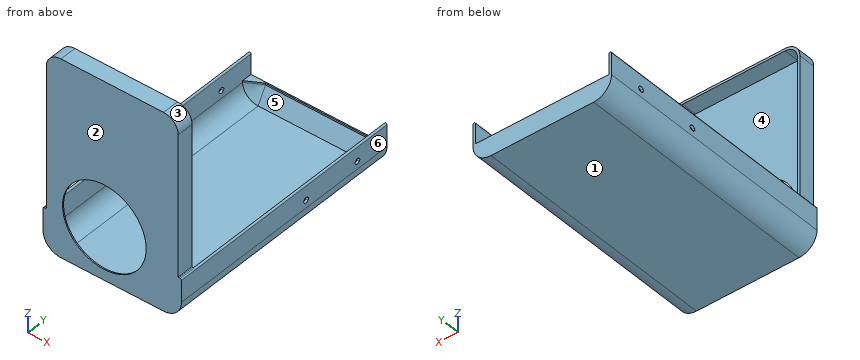
```python
from build123d import *
from OCP.BRepFilletAPI import BRepFilletAPI_MakeChamfer

# Parameters (mm, degrees)
BOSS_EXTRUDE1_DEPTH = 160
BOSS_EXTRUDE2_START = -0.8
BOSS_EXTRUDE2_DEPTH = 0.8
CUT_EXTRUDE1_DEPTH  = 185.952426316
SKETCH4_R           = 27
BOSS_EXTRUDE3_DEPTH = 0.8
FILLET1_R           = 0.4
BOSS_EXTRUDE4_DEPTH = 10
FILLET2_R           = 2
CHAMFER1_SIZE       = 5.7
CHAMFER1_SIZE2      = 9.872689603


with BuildPart() as part:
    # Sketch1 → Boss-Extrude1 (new body)
    with BuildSketch(Plane(origin=(0, 0, 0), x_dir=(1, 0, 0), z_dir=(0, 1, 0))):
        with BuildLine():
            Line((-33.1, 0), (33.1, 0))
            ThreePointArc((33.1, 0), (40.171067812, -2.928932188), (43.1, -10))
            Line((43.1, -10), (43.1, -24))
            ThreePointArc((43.1, -24), (43.9, -24.8), (44.7, -24))
            Line((44.7, -24), (44.7, -10))
            ThreePointArc((44.7, -10), (41.302438662, -1.797561338), (33.1, 1.6))
            Line((33.1, 1.6), (-33.1, 1.6))
            ThreePointArc((-33.1, 1.6), (-41.302438662, -1.797561338), (-44.7, -10))
            Line((-44.7, -10), (-44.7, -24))
            ThreePointArc((-44.7, -24), (-43.9, -24.8), (-43.1, -24))
            Line((-43.1, -24), (-43.1, -10))
            ThreePointArc((-43.1, -10), (-40.171067812, -2.928932188), (-33.1, 0))
        make_face()
    extrude(amount=BOSS_EXTRUDE1_DEPTH)

    # Sketch2 → Boss-Extrude2 (add)
    with BuildSketch(Plane(origin=(0, 160, 0), x_dir=(1, 0, 0), z_dir=(0, 1, 0)).offset(BOSS_EXTRUDE2_START)):
        with BuildLine():
            Line((44.7, -10), (44.7, -11))
            Line((44.7, -11), (-44.7, -11))
            Line((-44.7, -11), (-44.7, -10))
            ThreePointArc((-44.7, -10), (-41.302438662, -1.797561338), (-33.1, 1.6))
            Line((-33.1, 1.6), (33.1, 1.6))
            ThreePointArc((33.1, 1.6), (41.302438662, -1.797561338), (44.7, -10))
        make_face()
    extrude(amount=BOSS_EXTRUDE2_DEPTH)

    # Sketch3 → Cut-Extrude1 (cut, through all)
    with BuildSketch(Plane(origin=(44.7, 0, 0), x_dir=(0, 0, -1), z_dir=(1, 0, 0))):
        with BuildLine():
            Line((-15.875, 138.515544457), (-15, 139.020725942))
            Line((-15, 139.020725942), (-14.125, 138.515544457))
            ThreePointArc((-14.125, 138.515544457), (-13.25, 137), (-14.125, 135.484455543))
            Line((-14.125, 135.484455543), (-15, 134.979274058))
            Line((-15, 134.979274058), (-15.875, 135.484455543))
            ThreePointArc((-15.875, 135.484455543), (-16.75, 137), (-15.875, 138.515544457))
        make_face()
        with BuildLine():
            Line((-15.875, 98.515544457), (-15, 99.020725942))
            Line((-15, 99.020725942), (-14.125, 98.515544457))
            ThreePointArc((-14.125, 98.515544457), (-13.25, 97), (-14.125, 95.484455543))
            Line((-14.125, 95.484455543), (-15, 94.979274058))
            Line((-15, 94.979274058), (-15.875, 95.484455543))
            ThreePointArc((-15.875, 95.484455543), (-16.75, 97), (-15.875, 98.515544457))
        make_face()
    extrude(amount=-CUT_EXTRUDE1_DEPTH, mode=Mode.SUBTRACT)

    # Sketch4 → Boss-Extrude3 (add)
    with BuildSketch(Plane.XZ):
        with BuildLine():
            Line((-43.9, 24.8), (-42.6, 24.8))
            Line((-42.6, 24.8), (-42.6, 115.8))
            ThreePointArc((-42.6, 115.8), (-39.817514421, 122.517514421), (-33.1, 125.3))
            Line((-33.1, 125.3), (33.1, 125.3))
            ThreePointArc((33.1, 125.3), (39.817514421, 122.517514421), (42.6, 115.8))
            Line((42.6, 115.8), (42.6, 24.8))
            Line((42.6, 24.8), (43.9, 24.8))
            ThreePointArc((43.9, 24.8), (43.334314575, 24.565685425), (43.1, 24))
            Line((43.1, 24), (43.1, 10))
            ThreePointArc((43.1, 10), (40.171067812, 2.928932188), (33.1, 0))
            Line((33.1, 0), (-33.1, 0))
            ThreePointArc((-33.1, 0), (-40.171067812, 2.928932188), (-43.1, 10))
            Line((-43.1, 10), (-43.1, 24))
            ThreePointArc((-43.1, 24), (-43.334314575, 24.565685425), (-43.9, 24.8))
        make_face()
        with Locations(Location((-5.1, 32.3, 0), (0, 0, 270))):
            Circle(SKETCH4_R, mode=Mode.SUBTRACT)
    extrude(amount=-BOSS_EXTRUDE3_DEPTH)

    # Fillet1
    fillet1_edges = [part.edges().sort_by_distance(p)[0] for p in [
        (-42.6, 0.4, 24.8),
        (42.6, 0.4, 24.8),
    ]]
    fillet(fillet1_edges, radius=FILLET1_R)

    # Sketch6 → Boss-Extrude4 (add)
    with BuildSketch(Plane(origin=(0, 0.8, 0), x_dir=(1, 0, 0), z_dir=(0, 1, 0))):
        with BuildLine():
            Line((-43.1, -23.2), (-43, -23.2))
            ThreePointArc((-43, -23.2), (-41.585786438, -23.785786438), (-41, -25.2))
            Line((-41, -25.2), (-41, -115.8))
            ThreePointArc((-41, -115.8), (-38.686143571, -121.386143571), (-33.1, -123.7))
            Line((-33.1, -123.7), (33.1, -123.7))
            ThreePointArc((33.1, -123.7), (38.686143571, -121.386143571), (41, -115.8))
            Line((41, -115.8), (41, -25.2))
            ThreePointArc((41, -25.2), (41.585786438, -23.785786438), (43, -23.2))
            Line((43, -23.2), (43.1, -23.2))
            Line((43.1, -23.2), (43.1, -24))
            ThreePointArc((43.1, -24), (43.334314575, -24.565685425), (43.9, -24.8))
            Line((43.9, -24.8), (43, -24.8))
            ThreePointArc((43, -24.8), (42.717157288, -24.917157288), (42.6, -25.2))
            Line((42.6, -25.2), (42.6, -115.8))
            ThreePointArc((42.6, -115.8), (39.817514421, -122.517514421), (33.1, -125.3))
            Line((33.1, -125.3), (-33.1, -125.3))
            ThreePointArc((-33.1, -125.3), (-39.817514421, -122.517514421), (-42.6, -115.8))
            Line((-42.6, -115.8), (-42.6, -25.2))
            ThreePointArc((-42.6, -25.2), (-42.717157288, -24.917157288), (-43, -24.8))
            Line((-43, -24.8), (-43.9, -24.8))
            ThreePointArc((-43.9, -24.8), (-43.334314575, -24.565685425), (-43.1, -24))
            Line((-43.1, -24), (-43.1, -23.2))
        make_face()
    extrude(amount=BOSS_EXTRUDE4_DEPTH)

    # Fillet2
    # the kernel refuses this fillet: 2 mm, written as the material it adds along each edge
    with BuildSketch(Plane(origin=(43.1, 0.8, 23.2), x_dir=(-0.9748527767632401, 0, 0.22284986793130537), z_dir=(0, 1, 0))) as fillet2_piece_1:
        with BuildLine():
            CenterArc((1.610986416, -1.927420567), FILLET2_R, 105.482875224, 61.640649972)
            Line((-0.338719137, -1.481720831), (-0.533689693, -1.437150857))
            Line((-0.533689693, -1.437150857), (-0.194970555, 0.044569974))
            Line((-0.194970555, 0.044569974), (0.044569974, 0.194970555))
            ThreePointArc((0.044569974, 0.194970555), (0.142055251, 0.172685569), (1.023695645, 0.192742057))
            Line((1.023695645, 0.192742057), (1.077085715, 0))
        make_face()
    extrude(amount=10)
    with BuildSketch(Plane(origin=(-43.1, 0.8, 23.2), x_dir=(0.9748527767632457, 0, 0.2228498679312814), z_dir=(0, 1, 0))) as fillet2_piece_2:
        with BuildLine():
            CenterArc((1.610986416, 1.927420567), FILLET2_R, 192.876474804, 61.640649972)
            Line((-0.338719137, 1.481720831), (-0.533689693, 1.437150857))
            Line((-0.533689693, 1.437150857), (-0.194970555, -0.044569974))
            Line((-0.194970555, -0.044569974), (0.044569974, -0.194970555))
            ThreePointArc((0.044569974, -0.194970555), (0.142055251, -0.172685569), (1.023695645, -0.192742057))
            Line((1.023695645, -0.192742057), (1.077085715, 0))
        make_face()
    extrude(amount=10)

    # Chamfer1: one chamfer whose edges measure the first distance from different faces: ONE call of the kernel's chamfer builder (chamfer() names one face for all edges)
    chamfer1_edges_1 = [part.edges().sort_by_distance(p)[0] for p in [
        (0, 159.2, 0),
    ]]
    chamfer1_side_1 = [part.faces().sort_by_distance(p)[0] for p in [
        (0, 80, 0),
    ]]
    chamfer1_edges_2 = [part.edges().sort_by_distance(p)[0] for p in [
        (40.171067812, 159.2, 2.928932188),
    ]]
    chamfer1_side_2 = [part.faces().sort_by_distance(p)[0] for p in [
        (40.171067812, 80, 2.928932188),
    ]]
    chamfer1_edges_3 = [part.edges().sort_by_distance(p)[0] for p in [
        (43.1, 159.2, 10.5),
    ]]
    chamfer1_side_3 = [part.faces().sort_by_distance(p)[0] for p in [
        (43.1, 80.829745828, 16.958586697),
    ]]
    chamfer1_edges_4 = [part.edges().sort_by_distance(p)[0] for p in [
        (-43.1, 159.2, 10.5),
    ]]
    chamfer1_side_4 = [part.faces().sort_by_distance(p)[0] for p in [
        (-43.1, 80.829745828, 16.958586697),
    ]]
    chamfer1_edges_5 = [part.edges().sort_by_distance(p)[0] for p in [
        (-40.171067812, 159.2, 2.928932188),
    ]]
    chamfer1_side_5 = [part.faces().sort_by_distance(p)[0] for p in [
        (-40.171067812, 80, 2.928932188),
    ]]
    chamfer1 = BRepFilletAPI_MakeChamfer(part.part.solid().wrapped)
    for e in chamfer1_edges_1:
        chamfer1.Add(CHAMFER1_SIZE, CHAMFER1_SIZE2, e.wrapped, chamfer1_side_1[0].wrapped)  # the first distance lies on this face
    for e in chamfer1_edges_2:
        chamfer1.Add(CHAMFER1_SIZE, CHAMFER1_SIZE2, e.wrapped, chamfer1_side_2[0].wrapped)  # the first distance lies on this face
    for e in chamfer1_edges_3:
        chamfer1.Add(CHAMFER1_SIZE, CHAMFER1_SIZE2, e.wrapped, chamfer1_side_3[0].wrapped)  # the first distance lies on this face
    for e in chamfer1_edges_4:
        chamfer1.Add(CHAMFER1_SIZE, CHAMFER1_SIZE2, e.wrapped, chamfer1_side_4[0].wrapped)  # the first distance lies on this face
    for e in chamfer1_edges_5:
        chamfer1.Add(CHAMFER1_SIZE, CHAMFER1_SIZE2, e.wrapped, chamfer1_side_5[0].wrapped)  # the first distance lies on this face
    add(Compound.cast(chamfer1.Shape()), mode=Mode.REPLACE)


solid = part.part
```
CAD build for the part. Positions are in the model's coordinates, mm. Face numbers are marked on the shaded views. A direction names the side the tool comes from. Give positions to 0.01 mm unless a question says otherwise; leave off trailing zeros. Order: outer loops, then holes, each group sorted by start corner. A loop starts at its lowest first (then second) coordinate and runs counter-clockwise, first axis right, second up.
(1) Tool access for the marked faces 5 and 6: list every direction of +Z, -Z, +X, -X, +Y, -Y with a clear straight run to the whole face (end or side of a thin tool).
(2) Saw through at C-C, the plane z = 77. Give the cut face in (x, y), then the cut area to 3 significant figures.
(3) Saw through at B-B, the plane x = -5.1. Give the cut face in (y, z).
(4) Flat gauge pins, fed straight in: pin 1 (1.5 mm diameter, centred on x = 0, y = 45, fed in from +Z); pin 2 (5.5 mm diameter, centred on y = 6.5, z = 85, fed in from +X); pin 3 (5 mm diameter, centred on y = 4, z = 82, fed in from -X). Where does each tip first touch, or does it go through?
(5) Drill centre lines: L1, parallel to Z at x = 23.5, y = 9.5; L2, parallel to X at y = 0.65, z = 32.3; L3, parallel to X at y = 94, z = 18. Where is each one in solid material? Low to high.
(6) Mould opens along Z. For the marked faces 1, 2, 3 and 4 say: released by +Z, released by -Z, zero draft, split by the parting line, or undercut.
(7) Saw through at A-A, the plane z = 32.3. Give the cut face in (x, y), then the cut area to 3 significant figures.
(8) Saw through at D-D, the plane y = 47. Give the cut face in (x, z), then the cut area to 3 significant figures.
Results found:
1. face 5: +Z
1. face 6: +Z, -Z, +X, +Y, -Y
2. outline: (-42.6, 0) - (42.6, 0) - (42.6, 10.8) - (41, 10.8) - (41, 0.8) - (-41, 0.8) - (-41, 10.8) - (-42.6, 10.8) - close
2. area: 100 mm2
3. outline: (0, -1.6) - (160, -1.6) - (160, 11) - (159.2, 11) - (159.2, 9.87) - (153.5, 0) - (0.8, 0) - (0.8, 5.3) - (0, 5.3) - close; (0, 59.3) - (0.8, 59.3) - (0.8, 123.7) - (10.8, 123.7) - (10.8, 125.3) - (0, 125.3) - close
4. pin 1: stops at z = 0
4. pin 2: stops at x = 42.6
4. pin 3: stops at x = -42.6
5. L1: z = -1.6 to 0, 123.7 to 125.3
5. L2: x = -42.6 to -32.1, 21.9 to 42.6
5. L3: x = -44.7 to -43.1, 43.1 to 44.7
6. face 1: released by -Z
6. face 2: zero draft
6. face 3: released by +Z
6. face 4: undercut
7. outline: (-42.6, 0) - (-32.1, 0) - (-32.1, 0.8) - (-41, 0.8) - (-41, 10.8) - (-42.6, 10.8) - close; (21.9, 0) - (42.6, 0) - (42.6, 10.8) - (41, 10.8) - (41, 0.8) - (21.9, 0.8) - close
7. area: 57.0 mm2
8. outline: (-44.7, 10) arc R11.6 ccw to (-33.1, -1.6) - (33.1, -1.6) arc R11.6 ccw to (44.7, 10) - (44.7, 24) arc R0.8 ccw to (43.1, 24) - (43.1, 10) arc R10 cw to (33.1, 0) - (-33.1, 0) arc R10 cw to (-43.1, 10) - (-43.1, 24) arc R0.8 ccw to (-44.7, 24) - close
8. area: 207 mm2
